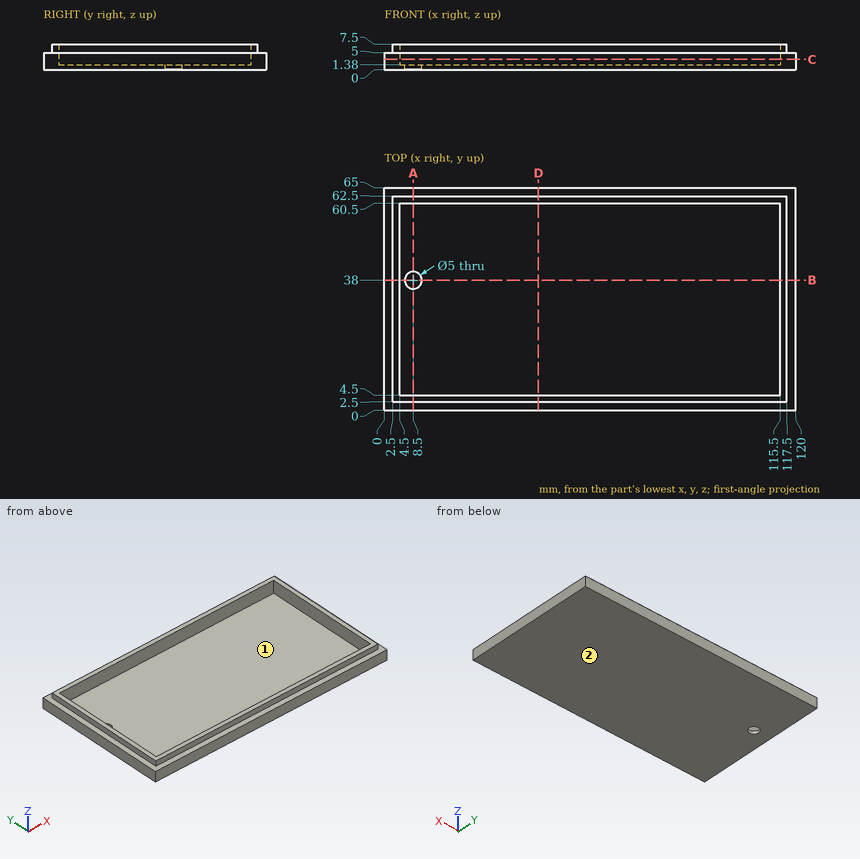
Geometry check sheet. Reference: drawing and pictorial views, mm from the part's lowest x, y, z. Round coordinates to 2 decimals unless told otherwise and drop trailing zeros. Order: outer loops, then holes, each group sorted by start corner. A loop starts at its lowest first (then second) coordinate and runs counter-clockwise, first axis right, second up.
Q1. Draft check along X on the marked faces 1 and 2. Enter one of: pulls with the +X half, pulls with the -X half, needs draft (parallel to the pull), parting line crosses it, or undercut.
Filled sheet:
face 1: undercut
face 2: needs draft
Q2. Cross-section at D-D, the plane x = 45. Enter the section's corners in (y, z), plus the area to 3 significant figures.
Filled sheet:
outline: (0, 0) - (65, 0) - (65, 5) - (62.5, 5) - (62.5, 7.5) - (60.5, 7.5) - (60.5, 1.38) - (4.5, 1.38) - (4.5, 7.5) - (2.5, 7.5) - (2.5, 5) - (0, 5) - close
area: 132 mm2
Q3. Cross-section at B-B, the plane y = 38. Enter the section's corners in (x, z), plus the area to 3 significant figures.
Filled sheet:
outline: (0, 0) - (6, 0) - (6, 1.38) - (4.5, 1.38) - (4.5, 7.5) - (2.5, 7.5) - (2.5, 5) - (0, 5) - close; (11, 0) - (120, 0) - (120, 5) - (117.5, 5) - (117.5, 7.5) - (115.5, 7.5) - (115.5, 1.38) - (11, 1.38) - close
area: 201 mm2
Q4. Depth check by flat-ended pin: P1, Ø3, axis at y = 38.5, z = 7, coming from the +X side; P2, Ø5, axis at x = 23, y = 11.5, coming from the +Z side; P3, Ø4.5, axis at x = 8.5, y = 38, coming from the -Z side. Enter the tip coordinate at first touch or a pass-through.
Filled sheet:
P1: stops at x = 117.5
P2: stops at z = 1.38
P3: passes through
Q5. Cross-section at A-A, the plane x = 8.5. Enter the section's corners in (y, z), plus the area to 3 significant figures.
Filled sheet:
outline: (0, 0) - (35.5, 0) - (35.5, 1.38) - (4.5, 1.38) - (4.5, 7.5) - (2.5, 7.5) - (2.5, 5) - (0, 5) - close; (40.5, 0) - (65, 0) - (65, 5) - (62.5, 5) - (62.5, 7.5) - (60.5, 7.5) - (60.5, 1.38) - (40.5, 1.38) - close
area: 125 mm2
Q6. Scan lines: L1, parallel to Y at x = 104, z = 2.25; L2, parallel to X at y = 8, z = 2.25; L3, parallel to X at y = 55, z = 5.5. Record each from-to range of solid material in increasing order.
Filled sheet:
L1: y = 0 to 4.5, 60.5 to 65
L2: x = 0 to 4.5, 115.5 to 120
L3: x = 2.5 to 4.5, 115.5 to 117.5
Q7. Cross-section at C-C, the plane z = 3. Enter the section's corners in (x, y), plus the area to 3 significant figures.
Filled sheet:
outline: (0, 0) - (120, 0) - (120, 65) - (0, 65) - close; hole (4.5, 4.5) - (115.5, 4.5) - (115.5, 60.5) - (4.5, 60.5) - close
area: 1,580 mm2
